The model under review builds one solid part; all positions refer to its coordinate system, in mm. A direction names the side the tool comes from. Round coordinates to 2 decimals unless told otherwise and drop trailing zeros. Loops run counter-clockwise (first coordinate to the right, second up) from the corner with the lowest first, then second, coordinate; pieces in that order, holes last. Notation, with made-up numbers: (70, 83) - (86, 83) arc R17 ccw to (86, 108) - close; hole circle Ø6 at (-24, 7.5). An arc over 180 degrees is marked (long way). Answer as CSV lines item,"result".
Autodesk Inventor part; units mm, degrees
ref_plane "YZ Plane" through (0, 0, 0) normal (1, 0, 0) x (0, 1, 0)
ref_plane "XZ Plane" through (0, 0, 0) normal (0, 1, 0) x (-1, 0, 0)
ref_plane "XY Plane" through (0, 0, 0) normal (0, 0, 1) x (1, 0, 0)
sketch "スケッチ1" plane through (0, 0, 0) normal (0, 0, 1) x (1, 0, 0)
  circle A0 centre (-56.2051, 45.5451) radius 2.75
  arc A1 (8.9566, 76.3281) -> (6.09, 76.7004) centre (7.222, 74.1942) ccw
  circle A2 centre (57.2805, 33.1812) radius 3
  line L0 (-57.3371, 48.0513) -> (6.09, 76.7004)
  line L1 (8.9566, 76.3281) -> (59.1728, 35.5091)
  line L2 (-57.6459, 48.7348) -> (5.7812, 77.3839)
  arc A3 (6.09, 76.7004) -> (8.9566, 76.3281) centre (7.222, 74.1942) ccw
  arc A4 (9.4296, 76.9101) -> (5.7812, 77.3839) centre (7.222, 74.1942) ccw
  line L3 (9.4296, 76.9101) -> (59.6459, 36.0911)
  line L4 (-57.6459, 48.7348) -> (-56.2051, 45.5451)
  line L5 (57.2805, 33.1812) -> (59.6459, 36.0911)
  line L6 (-53.0891, 50.793) -> (-52.7804, 50.1095)
  line L7 (55.2929, 38.663) -> (55.766, 39.2449)
  point P0 (0, 0)
  point P1 (5.7812, 77.3839)
  dimension "d0" = 0.75
  dimension "d1" = 0.75
  dimension "d2" = 0.75
  dimension "d3" = 5
  dimension "d4" = 5
extrude "押し出し1" add sketch "スケッチ1" along normal blind 30 contours L4 L2 L6 L0 | L6 L2 A4 L3 L7 L1 A1 L0
sketch "スケッチ2" plane through (-57.6459, 48.7348, 30) normal (-0.4116, 0.9113, 0) x (0.9113, 0.4116, 0)
  line L0 (69.5972, 30) -> (0, 30)
  line L1 (0, 30) -> (0, 0)
  line L2 (69.5972, 0) -> (0, 0)
  line L3 (69.5972, 30) -> (69.5972, 0)
  circle A0 centre (5, 15) radius 1.5
  point P0 (32.474, 30)
  dimension "d7" = 3
  dimension "d8" = 15
  dimension "d9" = 5
extrude "押し出し2" cut sketch "スケッチ2" against normal blind 0.75 contours A0
sketch "スケッチ3" plane through (9.4296, 76.9101, 30) normal (0.6308, 0.776, 0) x (0.776, -0.6308, 0)
  line L0 (59.7137, 30) -> (0, 30)
  line L1 (0, 30) -> (0, 0)
  line L2 (59.7137, 0) -> (0, 0)
  line L3 (59.7137, 30) -> (59.7137, 0)
  circle A0 centre (54.7137, 15) radius 1.5
  point P0 (41.1949, 30)
  dimension "d12" = 3
  dimension "d13" = 15
  dimension "d14" = 5
extrude "押し出し3" cut sketch "スケッチ3" against normal blind 0.75 contours A0
properties part number "クランクガード" material "ポリプロピレン"
1. Take a section at A-A (y = 60). State the section outline as (x, z) points, plus the area to 3 significant figures.
Numbers:
outline,"(-32.71, 0) - (-30.88, 0) - (-30.88, 30) - (-32.71, 30) - close; (29.04, 0) - (30.23, 0) - (30.23, 30) - (29.04, 30) - close"
area,"90.3 mm²"
2. Tool access review of faces 4 (the face through (32.273, 58.341, 14.79)), 5 (the face through (31.8, 57.76, 14.79)): name each direction out of +Z, -Z, +X, -X, +Y, -Y from which nothing blocks a thin tool from reaching the whole face with its end or side.
Numbers:
face 4,"+Z, -Z, +X, +Y"
face 5,"+Z, -Z, -Y"
3. Draft analysis for pull direction X (two halves, no side actions). For faces 1 (the face through (7.555, 76.924, 14.79)), 2 (the face through (-1, 74, 30)), 3 (the face through (7.646, 77.668, 14.79)), state which applies: +X half, -X half, draft (parallel to the pull), parting line (faces both ways), or undercut.
Numbers:
face 1,"undercut"
face 2,"draft"
face 3,"parting line"
4. Take a section at C-C (z = 24.5). State the section outline as (x, y) points.
Numbers:
outline,"(-57.65, 48.73) - (-57.34, 48.05) - (6.09, 76.7) arc R2.75 cw to (8.96, 76.33) - (55.29, 38.66) - (55.77, 39.24) - (9.43, 76.91) arc R3.5 ccw to (5.78, 77.38) - close"
5. Take a section at B-B (y = 73.5). State the section outline as (x, z) points.
Numbers:
outline,"(-2.82, 0) - (-1, 0) - (-1, 30) - (-2.82, 30) - close; (12.44, 0) - (13.62, 0) - (13.62, 30) - (12.44, 30) - close"
6. Wall thickness on probe 1 along X at (y, z) = (75, 11); probe 2 along X at (y, z) = (51, 6.5); probe 3 along Y at (x, z) = (-23, 16): over which ranges is each line inside the solid? List them lowest first.
Numbers:
probe 1,"x = 0.5 to 2.33, 10.59 to 11.78"
probe 2,"x = -52.63 to -50.81, 40.12 to 41.3"
probe 3,"y = 63.56 to 64.38"
7. Clearance check with flat-ended pins moving along their axes: pin 1 (5 mm diameter, centred on y = 56, z = 24, fed in from -X); pin 2 (12 mm diameter, centred on x = -46, z = 12, fed in from +Y); pin 3 (5 mm diameter, centred on x = 35.5, z = 16, fed in from +Y); pin 4 (10 mm diameter, centred on x = 21, y = 59.5, fed in from -Z). State where each tip first meets the part, or that it passes through.
Numbers:
pin 1,"stops at x = -47.1"
pin 2,"stops at y = 56.71"
pin 3,"stops at y = 57.75"
pin 4,"passes through"
8. Take a section at D-D (x = -18.5). State the section outline as (y, z) points.
Numbers:
outline,"(65.59, 0) - (66.42, 0) - (66.42, 30) - (65.59, 30) - close"
